from build123d import *

# Parameters (mm, degrees)
SKETCH_R  = 2.1
PAD_DEPTH = 100


with BuildPart() as part:
    # Sketch → Pad (new body)
    with BuildSketch(Plane.XY):
        Polygon((0, -3.691567), (0.174924, -3.891567), (2.84, -3.891567), (5.535042, -6.586609), (5.535042, -8.2), (3.1, -8.2), (4.9, -10), (10, -10), (10, -4.9), (8.2, -3.1), (8.2, -5.535042), (6.586609, -5.535042), (3.891567, -2.84), (3.891567, -0.174924), (3.691567, 0), (3.891567, 0.170281), (3.891567, 2.84), (6.576242, 5.524674), (8.2, 5.524674), (8.2, 3.1), (10, 4.9), (10, 10), (4.9, 10), (3.1, 8.2), (5.524674, 8.2), (5.524674, 6.576242), (2.84, 3.891567), (0.170281, 3.891567), (0, 3.691567), (-0.219864, 3.891567), (-2.84, 3.891567), (-5.490619, 6.542187), (-5.490619, 8.2), (-3.1, 8.2), (-4.9, 10), (-10, 10), (-10, 4.9), (-8.2, 3.1), (-8.2, 5.490619), (-6.542187, 5.490619), (-3.891567, 2.84), (-3.891567, 0.219864), (-3.691567, 0), (-3.891567, -0.224285), (-3.891567, -2.84), (-6.587748, -5.53618), (-8.2, -5.53618), (-8.2, -3.1), (-10, -4.9), (-10, -10), (-4.9, -10), (-3.1, -8.2), (-5.53618, -8.2), (-5.53618, -6.587748), (-2.84, -3.891567), (-0.224285, -3.891567), align=None)
        Circle(SKETCH_R, mode=Mode.SUBTRACT)
    extrude(amount=PAD_DEPTH)


solid = part.part
Model file for the job. Use its own axes, mm. A direction names the side the tool comes from. Round coordinates to 2 decimals unless told otherwise and drop trailing zeros.
1. Wall check: probe 1 along Y at (x, z) = (0, 54); probe 2 along X at (y, z) = (-7.5, 71); probe 3 along Y at (x, z) = (7, 86.5). Give the ranges that are in metal, low to high.
Check values:
probe 1: y = -3.69 to -2.1, 2.1 to 3.69
probe 2: x = -10 to -5.54, 5.54 to 10
probe 3: y = -10 to -5.54, 5.52 to 10
2. Drop flat-ended pins along their axis: P1, Ø0.7, axis at y = -4.5, z = 61.5, coming from the -X side; P2, Ø0.7, axis at x = -3.5, z = 36, coming from the +Y side; P3, Ø0.8, axis at y = -1, z = 34, coming from the -X side. Give the stop position or say it passes through.
Check values:
P1: stops at x = -9.95
P2: stops at y = 8.95
P3: stops at x = -3.89
3. Tool access for faces 4 (the flat face through (9.1, 4, 49.3)), 5 (the flat face through (-9.1, -4, 49.3)), 6 (the flat face through (1, -3.892, 49)), 7 (the flat face through (-4, 9.1, 49.3)), 8 (the flat face through (-7, 5.491, 49)): list every direction of +Z, -Z, +X, -X, +Y, -Y with a clear straight run to the whole face (end or side of a thin tool).
Check values:
face 4: +Z, -Z, +X
face 5: +Z, -Z, -X
face 6: +Z, -Z, -Y
face 7: +Z, -Z, +Y
face 8: +Z, -Z
4. Mould opens along X. For faces 1 (the flat face through (4, -9.1, 49.3)), 2 (the flat face through (-7, 10, 49)), 3 (the flat face through (3.892, -2, 49)) say: +X half, -X half, draft (parallel to the pull), parting line (faces both ways), or undercut.
Check values:
face 1: undercut
face 2: draft
face 3: +X half
